Geometry: final body of the model. Coordinates: model frame, mm. Coordinates: 2 decimals unless noted, no trailing zeros. Write each loop counter-clockwise with the first axis right and the second up, starting at its lowest first coordinate (ties: lowest second). Pieces come first, ordered by that corner, then holes. Notation, with made-up numbers: (-5.75, -20) - (50.25, -20) arc R26 cw to (50.25, 17) - close; hole circle Ø7 at (0, 47). An arc over 180 degrees is marked (long way). Answer as a JSON object with one key per item and string values. Group by question number.
Item 1: Section B-B on x = 1622. Return loops of the section in (y, z), and give its area (3 significant figures).
Item 2: Line query: line 1 along Z through (x, y) = (389, -25.4); line 2 along Y through (x, z) = (2155, 36.5); line 3 along Z through (x, y) = (1857.5, -30). Output: solid intervals per line, ascending. Write a range as from..to.
Item 3: Section A-A on y = -27. Return loops of the section in (x, z).
Item 4: First-contact query: pin 1 Ø2 at (y, z) = (-22, -6.5) entering from +X; pin 2 Ø6 at (x, z) = (1603.5, -12.5) entering from +Y; pin 3 Ø4 at (y, z) = (-41, 45) entering from +X. Flat tips, straight axial feed; report the tip coordinate or a pass-through.
```python
from build123d import *

# Parameters (mm, degrees)
F0_W        = 2540
F0_H        = 152.4
F1_DEPTH    = 50.8
F2_R        = 12.7
F3_DEPTH    = 2540
F4_T1_DEPTH = 413.6829915773


# Not quite as in the source:
# - a fillet or chamfer that OpenCascade refuses, or shapes differently, is made with other operations: its cross-section is extruded or revolved along the edge and cut away or added


with BuildPart() as f1:
    # F0 (on Front) → F1 (new body)
    with BuildSketch(Plane.XZ):
        with Locations((996.8233792729, 9.1693531722)):
            Rectangle(F0_W, F0_H)
    extrude(amount=F1_DEPTH)

    # F2 (on face) → F3 (cut)
    with BuildSketch(Plane(origin=(-273.1766207271, 0, 0), x_dir=(0, -1, 0), z_dir=(-1, 0, 0))):
        with Locations((25.4, 34.5693531722)):
            Circle(F2_R)
        with Locations((25.4, -16.2306468278)):
            Circle(F2_R)
    extrude(amount=-F3_DEPTH, mode=Mode.SUBTRACT)

    # F4: chamfer of 50.8 on 1 edges, made by hand

    # F4_s2 → F4_t1 (cut)
    with BuildSketch(Plane.XY.offset(-197.6721426165)):
        Polygon((2266.8233792729, -50.8), (2216.0233792729, 0), (2266.8233792729, 0), align=None)
    extrude(amount=F4_T1_DEPTH, mode=Mode.SUBTRACT)


solid = f1.part
```
Checks:
{
 "1": {"outline": "(-50.8, -67.03) - (0, -67.03) - (0, 85.37) - (-50.8, 85.37) - close; hole circle Ø25.4 at (-25.4, -16.23); hole circle Ø25.4 at (-25.4, 34.57)", "area": "6,730 mm^2"},
 "2": {"line 1": "-67.03..-28.93, -3.53..21.87, 47.27..85.37", "line 2": "-50.8..-37.95, -12.85..0", "line 3": "-67.03..-28.07, -4.39..22.73, 46.41..85.37"},
 "3": {"outline": "(-273.18, -67.03) - (2243.02, -67.03) - (2243.02, -28.83) - (-273.18, -28.83) - close; (-273.18, -3.63) - (2243.02, -3.63) - (2243.02, 21.97) - (-273.18, 21.97) - close; (-273.18, 47.17) - (2243.02, 47.17) - (2243.02, 85.37) - (-273.18, 85.37) - close"},
 "4": {"pin 1": "through", "pin 2": "y = 0", "pin 3": "x = 2259.02"}
}
